Design review of the part built by this model. Coordinates are the model's own, in mm. Round coordinates to 2 decimals unless told otherwise and drop trailing zeros. One line per question, with ' | ' between items. Start each with the question number.
Item 1: Add section A-A, the plane y = -295.5. Give the number of separate pieces and of enclosed holes in the cut face, and give its area (3 significant figures).
Item 2: For L1, parallel to X at y = -445, z = -4.5; L2, parallel to Z at x = -7, y = -256.5; L3, parallel to Z at x = 0, y = -217, list the stretches that pass through material, from the lowest coordinate up.
Item 3: Insertion check: pin 1 Ø2 at (y, z) = (-395.5, -2.5) entering from +X; pin 2 Ø0.8 at (y, z) = (-242.5, 4) entering from +X; pin 3 Ø6 at (x, y) = (-1, -287.5) entering from +Z. Each pin has a flat end and moves straight along its axis. Give the tip position at first contact, or say it passes through.
```python
from build123d import *

# Parameters (mm, degrees)
F0_W            = 20
F0_H            = 20
F1_DEPTH        = 503
F2_R            = 2.1
F3_DEPTH        = 503.001
F4_R            = 1
F6_DEPTH        = 503.001
F6_COPIES_COUNT = 4


# Not quite as in the source:
# - a pattern or mirror of a feature is missing from the dataset's text; its kind, count and spacing are read off the source's solid


with BuildPart() as f1:
    # F0 (on Front) → F1 (new body)
    with BuildSketch(Plane.XZ):
        Rectangle(F0_W, F0_H)
    extrude(amount=F1_DEPTH)

    # F2 (on face) → F3 (cut, through all)
    with BuildSketch(Plane.XZ.offset(503)):
        Circle(F2_R)
    extrude(amount=-F3_DEPTH, mode=Mode.SUBTRACT)

    # F4
    f4_edges = [f1.edges().sort_by_distance(p)[0] for p in [
        (-10, -251.5, 10),
        (10, -251.5, 10),
        (10, -251.5, -10),
        (-10, -251.5, -10),
    ]]
    fillet(f4_edges, radius=F4_R)

    # F5 (on face) → F6 (cut, through all)
    with BuildSketch(Plane.XZ.offset(503)):
        Polygon((0, 3.9006601718), (0, 10), (-2.84, 10), (-4.64, 10), (-2.84, 8.2), (-5.4993398282, 8.2), (-5.4993398282, 6.56), (-2.84, 3.9006601718), align=None)
        Polygon((-6.5693398282, 8.2), (-8.2, 8.2), (-7.0953059148, 7.0953059148), (-6.5693398282, 7.6212720014), align=None)
    f6 = extrude(amount=-F6_DEPTH, mode=Mode.SUBTRACT)

    # F6_copies: F6 ×4 about axis
    f6_copies_axis = Axis((0, 0, 0), (0, 1, 0))
    for i in range(1, F6_COPIES_COUNT):
        add(f6.rotate(f6_copies_axis, i * 360 / F6_COPIES_COUNT), mode=Mode.SUBTRACT)

    # F6_copies1: F6 across plane
    add(f6.mirror(Plane(origin=(0, 0, 0), x_dir=(-0.7071067812, 0, -0.7071067812), z_dir=(0.7071067812, 0, -0.7071067812))), mode=Mode.SUBTRACT)

    # F6_copies2: F6 across plane
    add(f6.mirror(Plane(origin=(0, 0, 0), x_dir=(-1, 0, 0), z_dir=(0, 0, -1))), mode=Mode.SUBTRACT)

    # F6_copies3: F6 across plane
    add(f6.mirror(Plane(origin=(0, 0, 0), x_dir=(0, 0, 1), z_dir=(1, 0, 0))), mode=Mode.SUBTRACT)

    # F6_copies4: F6 across plane
    add(f6.mirror(Plane(origin=(0, 0, 0), x_dir=(0.7071067812, 0, -0.7071067812), z_dir=(-0.7071067812, 0, -0.7071067812))), mode=Mode.SUBTRACT)


solid = f1.part
```
Computed values:
1) separate pieces: 1 | enclosed holes: 5 | area: 162 mm^2
2) L1: x = -9.86 to -8.2, -5.56 to -3.44, 3.44 to 5.56, 8.2 to 9.86 | L2: z = -10 to -8.2, -7.19 to -5.5, 5.5 to 7.19, 8.2 to 10 | L3: z = -3.9 to -2.1, 2.1 to 3.9
3) pin 1: stops at x = 8.86 | pin 2: stops at x = 9.76 | pin 3: stops at z = 9.36
